```python
from build123d import *

# Parameters (mm, degrees)
F1_DEPTH     = 63.5
F0_W         = 25.4
F0_H         = 19.05
F2_DEPTH     = 12.7
F3_DEPTH     = 7.9375
F5_R         = 6.35
F6_T1_DEPTH  = 114.3
F6_T3_DEPTH  = 17.4752
F6_T5_DEPTH  = 49.2125
F6_T7_DEPTH  = 69.85
F6_T9_DEPTH  = 44.45
F6_T12_ANGLE = 90
F6_T14_ANGLE = 90
F6_T16_ANGLE = 90
F6_T18_ANGLE = 90
F6_T20_ANGLE = 90
F6_T22_ANGLE = 90
F6_T26_DEPTH = 19.2779547439
F6_S27_R     = 25.4
F6_T28_DEPTH = 12
F6_T30_ANGLE = 90
F6_T35_DEPTH = 57.15
F6_T39_DEPTH = 30.1752


# Not quite as in the source:
# - a fillet or chamfer that OpenCascade refuses, or shapes differently, is made with other operations: its cross-section is extruded or revolved along the edge and cut away or added


with BuildPart() as f1:
    # F0 (on Front) → F1 (new body, symmetric)
    with BuildSketch(Plane.XZ):
        Polygon((-41.275, 9.525), (-41.275, -9.525), (41.275, -9.525), (41.275, 9.525), (22.225, 9.525), align=None)
    extrude(amount=F1_DEPTH, both=True)

    # F0 (on Front) → F2 (join, symmetric)
    with BuildSketch(Plane.XZ):
        with BuildLine():
            Line((22.225, 9.525), (41.275, 9.525))
            Line((41.275, 9.525), (41.275, 27.0002))
            ThreePointArc((41.275, 27.0002), (45.9246798487, 38.2255201513), (57.15, 42.8752))
            Line((57.15, 42.8752), (60.325, 42.8752))
            Line((60.325, 42.8752), (60.325, 61.9252))
            Line((60.325, 61.9252), (57.15, 61.9252))
            add(Edge.make_bspline(
                [(52.2120910402, 61.5743620304), (53.8564284602, 61.7203088284), (55.5029986104, 61.8377030625), (57.15, 61.9252)],
                knots=[107.7945152041, 107.7945152041, 107.7945152041, 107.7945152041, 111.5045361635, 111.5045361635, 111.5045361635, 111.5045361635], degree=3))
            ThreePointArc((52.2120910402, 61.5743620304), (30.766178296, 49.8835908608), (22.225, 27.0002))
            Line((22.225, 27.0002), (22.225, 9.525))
        make_face()
        with Locations((73.025, 52.4002)):
            Rectangle(F0_W, F0_H)
    extrude(amount=F2_DEPTH, both=True)

    # F0 (on Front) → F3 (join, symmetric)
    with BuildSketch(Plane.XZ):
        with BuildLine():
            add(Edge.make_bspline(
                [(-41.275, 9.525), (-41.4553787608, 28.9895938663), (4.4359310246, 57.3338834698), (52.2120910402, 61.5743620304)],
                knots=[0, 0, 0, 0, 107.7945152041, 107.7945152041, 107.7945152041, 107.7945152041], degree=3))
            Line((-41.275, 9.525), (22.225, 9.525))
            Line((22.225, 9.525), (22.225, 27.0002))
            ThreePointArc((22.225, 27.0002), (30.766178296, 49.8835908608), (52.2120910402, 61.5743620304))
        make_face()
    extrude(amount=F3_DEPTH, both=True)

    # F0 (on Front) → F4 (revolve)
    with BuildSketch(Plane.XZ):
        Polygon((85.725, 66.675), (85.725, 61.9252), (85.725, 42.8752), (85.725, 38.1), (111.125, 38.1), (111.125, 66.675), align=None)
    revolve(axis=Axis((85.725, 0, 52.3875), (0, 0, -1)))

    # F5
    f5_edges = [f1.edges().sort_by_distance(p)[0] for p in [
        (41.275, -63.5, 0),
        (-41.275, -63.5, 0),
        (41.275, 63.5, 0),
        (-41.275, 63.5, 0),
    ]]
    fillet(f5_edges, radius=F5_R)

    # F6: fillet of radius 5.08 on 16 edges, made by hand

    # F6_s2 → F6_t1 (cut)
    with BuildSketch(Plane.XZ.offset(-57.15)):
        with BuildLine():
            ThreePointArc((36.195, -9.525), (39.7871024484, -8.0371024484), (41.275, -4.445))
            Line((41.275, -4.445), (41.275, -9.525))
            Line((41.275, -9.525), (36.195, -9.525))
        make_face()
        with BuildLine():
            ThreePointArc((-41.275, -4.445), (-39.7871024484, -8.0371024484), (-36.195, -9.525))
            Line((-36.195, -9.525), (-41.275, -9.525))
            Line((-41.275, -9.525), (-41.275, -4.445))
        make_face()
    extrude(amount=F6_T1_DEPTH, mode=Mode.SUBTRACT)

    # F6_s4 → F6_t3 (cut)
    with BuildSketch(Plane.XY.offset(9.525)):
        with BuildLine():
            ThreePointArc((41.275, -7.62), (39.7871024484, -11.2121024484), (36.195, -12.7))
            Line((36.195, -12.7), (41.275, -12.7))
            Line((41.275, -12.7), (41.275, -7.62))
        make_face()
    extrude(amount=F6_T3_DEPTH, mode=Mode.SUBTRACT)

    # F6_s6 → F6_t5 (cut)
    with BuildSketch(Plane.XZ.offset(7.9375)):
        with BuildLine():
            ThreePointArc((-41.275, 4.445), (-39.7871024484, 8.0371024484), (-36.195, 9.525))
            Line((-36.195, 9.525), (-41.275, 9.525))
            Line((-41.275, 9.525), (-41.275, 4.445))
        make_face()
    extrude(amount=F6_T5_DEPTH, mode=Mode.SUBTRACT)

    # F6_s8 → F6_t7 (cut)
    with BuildSketch(Plane.YZ.offset(-34.925)):
        with BuildLine():
            ThreePointArc((58.42, -9.525), (62.0121024484, -8.0371024484), (63.5, -4.445))
            Line((63.5, -4.445), (63.5, -9.525))
            Line((63.5, -9.525), (58.42, -9.525))
        make_face()
        with BuildLine():
            ThreePointArc((-58.42, -9.525), (-62.0121024484, -8.0371024484), (-63.5, -4.445))
            Line((-63.5, -4.445), (-63.5, -9.525))
            Line((-63.5, -9.525), (-58.42, -9.525))
        make_face()
        with BuildLine():
            ThreePointArc((-58.42, 9.525), (-62.0121024484, 8.0371024484), (-63.5, 4.445))
            Line((-63.5, 4.445), (-63.5, 9.525))
            Line((-63.5, 9.525), (-58.42, 9.525))
        make_face()
    extrude(amount=F6_T7_DEPTH, mode=Mode.SUBTRACT)

    # F6_s10 → F6_t9 (cut)
    with BuildSketch(Plane.XZ.offset(12.7)):
        with BuildLine():
            ThreePointArc((36.195, 9.525), (39.7871024484, 8.0371024484), (41.275, 4.445))
            Line((41.275, 4.445), (41.275, 9.525))
            Line((41.275, 9.525), (36.195, 9.525))
        make_face()
    extrude(amount=F6_T9_DEPTH, mode=Mode.SUBTRACT)

    # F6_s11 → F6_t12 (revolve, cut)
    with BuildSketch(Plane.YZ.offset(34.925)):
        with BuildLine():
            ThreePointArc((-58.42, 9.525), (-62.0121024484, 8.0371024484), (-63.5, 4.445))
            Line((-63.5, 4.445), (-63.5, 9.525))
            Line((-63.5, 9.525), (-58.42, 9.525))
        make_face()
    revolve(axis=Axis((34.925, -57.15, 9.525), (0, 0, 1)), revolution_arc=F6_T12_ANGLE, mode=Mode.SUBTRACT)

    # F6_s13 → F6_t14 (revolve, cut)
    with BuildSketch(Plane.XZ.offset(-57.15)):
        with BuildLine():
            ThreePointArc((-36.195, -9.525), (-39.7871024484, -8.0371024484), (-41.275, -4.445))
            Line((-41.275, -4.445), (-41.275, -9.525))
            Line((-41.275, -9.525), (-36.195, -9.525))
        make_face()
    revolve(axis=Axis((-34.925, 57.15, -9.525), (0, 0, -1)), revolution_arc=F6_T14_ANGLE, mode=Mode.SUBTRACT)

    # F6_s15 → F6_t16 (revolve, cut)
    with BuildSketch(Plane.XZ.offset(57.15)):
        with BuildLine():
            ThreePointArc((-36.195, -9.525), (-39.7871024484, -8.0371024484), (-41.275, -4.445))
            Line((-41.275, -4.445), (-41.275, -9.525))
            Line((-41.275, -9.525), (-36.195, -9.525))
        make_face()
    revolve(axis=Axis((-34.925, -57.15, -9.525), (0, 0, 1)), revolution_arc=F6_T16_ANGLE, mode=Mode.SUBTRACT)

    # F6_s17 → F6_t18 (revolve, cut)
    with BuildSketch(Plane.YZ.offset(34.925)):
        with BuildLine():
            ThreePointArc((58.42, -9.525), (62.0121024484, -8.0371024484), (63.5, -4.445))
            Line((63.5, -4.445), (63.5, -9.525))
            Line((63.5, -9.525), (58.42, -9.525))
        make_face()
    revolve(axis=Axis((34.925, 57.15, -9.525), (0, 0, -1)), revolution_arc=F6_T18_ANGLE, mode=Mode.SUBTRACT)

    # F6_s19 → F6_t20 (revolve, cut)
    with BuildSketch(Plane.YZ.offset(34.925)):
        with BuildLine():
            ThreePointArc((-58.42, -9.525), (-62.0121024484, -8.0371024484), (-63.5, -4.445))
            Line((-63.5, -4.445), (-63.5, -9.525))
            Line((-63.5, -9.525), (-58.42, -9.525))
        make_face()
    revolve(axis=Axis((34.925, -57.15, -9.525), (0, 0, 1)), revolution_arc=F6_T20_ANGLE, mode=Mode.SUBTRACT)

    # F6_s21 → F6_t22 (revolve, cut)
    with BuildSketch(Plane.XZ.offset(57.15)):
        with BuildLine():
            ThreePointArc((-41.275, 4.445), (-39.7871024484, 8.0371024484), (-36.195, 9.525))
            Line((-36.195, 9.525), (-41.275, 9.525))
            Line((-41.275, 9.525), (-41.275, 4.445))
        make_face()
    revolve(axis=Axis((-34.925, -57.15, 9.525), (0, 0, 1)), revolution_arc=F6_T22_ANGLE, mode=Mode.SUBTRACT)


with BuildPart() as f6_tool24:
    # F6_s25 → F6_t26 (new body)
    with BuildSketch(Plane.YZ.offset(57.15)):
        with BuildLine():
            ThreePointArc((-12.7, 47.9552), (-11.2121024484, 44.3630975516), (-7.62, 42.8752))
            Line((-7.62, 42.8752), (-12.7, 42.8752))
            Line((-12.7, 42.8752), (-12.7, 47.9552))
        make_face()
    extrude(amount=F6_T26_DEPTH)

    # F6_s27 → F6_t28 (cut, symmetric)
    with BuildSketch(Plane.XY.offset(45.4)):
        with Locations((85.725, 0)):
            Circle(F6_S27_R)
    extrude(amount=F6_T28_DEPTH, both=True, mode=Mode.SUBTRACT)


with BuildPart() as f1_1:
    add(f1.part)

    # F6_t23: cut F6_tool24
    add(f6_tool24.part, mode=Mode.SUBTRACT)

    # F6_s29 → F6_t30 (revolve, cut)
    with BuildSketch(Plane.XY.offset(27.0002)):
        with BuildLine():
            ThreePointArc((36.195, -12.7), (39.7871024484, -11.2121024484), (41.275, -7.62))
            Line((41.275, -7.62), (41.275, -12.7))
            Line((41.275, -12.7), (36.195, -12.7))
        make_face()
    revolve(axis=Axis((57.15, -12.7, 27.0002), (0, 1, 0)), revolution_arc=F6_T30_ANGLE, mode=Mode.SUBTRACT)


with BuildPart() as f6_tool33:
    # F6_s34 → F6_t35 (new body)
    with BuildSketch(Plane.XZ.offset(57.15)):
        with BuildLine():
            ThreePointArc((36.195, 9.525), (39.7871024484, 8.0371024484), (41.275, 4.445))
            Line((41.275, 4.445), (41.275, 9.525))
            Line((41.275, 9.525), (36.195, 9.525))
        make_face()
    extrude(amount=-F6_T35_DEPTH)

    split(bisect_by=Plane.XZ.offset(12.7), keep=Keep.BOTTOM)


with BuildPart() as f6_tool37:
    # F6_s38 → F6_t39 (new body)
    with BuildSketch(Plane.XY.offset(-3.175)):
        with BuildLine():
            ThreePointArc((41.275, -7.62), (39.7871024484, -11.2121024484), (36.195, -12.7))
            Line((36.195, -12.7), (41.275, -12.7))
            Line((41.275, -12.7), (41.275, -7.62))
        make_face()
    extrude(amount=F6_T39_DEPTH)

    split(bisect_by=Plane.XY.offset(9.525), keep=Keep.BOTTOM)


with BuildPart() as f6_tool33_1:
    add(f6_tool33.part)

    # F6_t41: intersect F6_tool37
    add(f6_tool37.part, mode=Mode.INTERSECT)


with BuildPart() as f1_2:
    add(f1_1.part)

    # F6_t31: cut F6_tool33
    add(f6_tool33_1.part, mode=Mode.SUBTRACT)


solid = f1_2.part
```
The model under review builds one solid part; all positions refer to its coordinate system, in mm. A direction names the side the tool comes from. Round coordinates to 2 decimals unless told otherwise and drop trailing zeros. Loops run counter-clockwise (first coordinate to the right, second up) from the corner with the lowest first, then second, coordinate; pieces in that order, holes last.
Item 1: For line 1 (Z direction, x = -18, y = 44) (3 decimals); line 2 (Y direction, x = 21.5, z = 31); line 3 (Z direction, x = 101.5, y = -12) (3 decimals), list the stretches that pass through material, from the lowest coordinate up.
Determined:
line 1: z = -9.525 to 9.525
line 2: y = -7.94 to 7.94
line 3: z = 38.1 to 66.675
Item 2: Mouldability with a two-part tool opening along Z and no side actions: class faces 1 (the face through (86, 0, 38.1)), 2 (the face through (-39.826, -32.199, 7.997)), 3 (the face through (39.8, -11.2, 18.1)), 4 (the face through (22.225, 10, 18)) as released by +Z, released by -Z, zero draft, split by the parting line, or undercut.
Determined:
face 1: released by -Z
face 2: released by +Z
face 3: undercut
face 4: zero draft
Item 3: Clearance check with flat-ended pins moving along their axes: pin 1 Ø2 at (x, y) = (75.5, 20) entering from -Z; pin 2 Ø15.5 at (x, z) = (7.5, 47) entering from +Y; pin 3 Ø4 at (x, y) = (46.5, 9) entering from +Z. State where each tip first meets the part, or that it passes through.
Determined:
pin 1: stops at z = 38.1
pin 2: stops at y = 7.94
pin 3: stops at z = 61.16
Item 4: Take a section at A-A (y = 21). Write out the cut boundary in (x, z) (3 decimals), then the cut area to 3 significant figures.
Determined:
outline: (-41.275, -4.445) arc R5.08 ccw to (-36.195, -9.525) - (36.195, -9.525) arc R5.08 ccw to (41.275, -4.445) - (41.275, 9.525) - (-41.275, 9.525) - close; (71.437, 38.1) - (100.013, 38.1) - (100.013, 66.675) - (71.437, 66.675) - close
area: 2,380 mm2
Item 5: Take a section at C-C (y = -37). Write out the cut boundary in (x, z) (3 decimals).
Determined:
outline: (-41.275, -4.445) arc R5.08 ccw to (-36.195, -9.525) - (36.195, -9.525) arc R5.08 ccw to (41.275, -4.445) - (41.275, 4.445) arc R5.08 ccw to (36.195, 9.525) - (-36.195, 9.525) arc R5.08 ccw to (-41.275, 4.445) - close
Item 6: Take a section at B-B (y = 37.5). Write out the cut boundary in (x, z) (3 decimals).
Determined:
outline: (-41.275, -4.445) arc R5.08 ccw to (-36.195, -9.525) - (36.195, -9.525) arc R5.08 ccw to (41.275, -4.445) - (41.275, 9.525) - (-41.275, 9.525) - close
Item 7: For faces 5 (the face through (0, 63.5, 3)), 6 (the face through (-4, -7.938, 33)), list the 3-axis set-ups (+Z, -Z, +X, -X, +Y, -Y) from which the entire face can be reached by the end or side of a thin tool; tool diameter is ignored.
Determined:
face 5: +Z, -Z, +X, -X, +Y
face 6: +Z, -X, -Y
Item 8: Take a section at D-D (x = 70). Write out the cut boundary in (y, z) (3 decimals).
Determined:
outline: (-19.947, 38.1) - (19.947, 38.1) - (19.947, 66.675) - (-19.947, 66.675) - close
